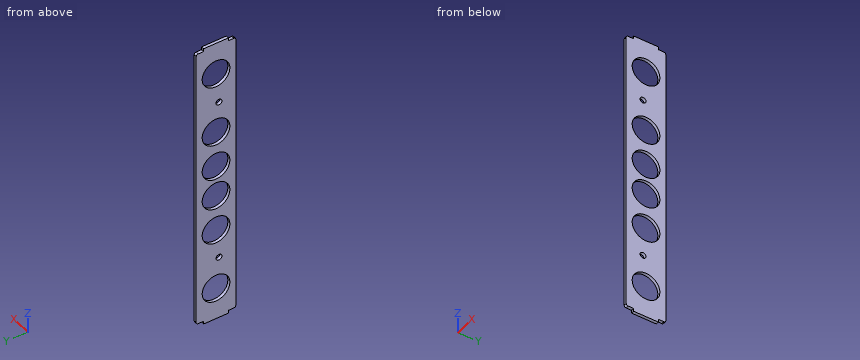
```python
from build123d import *

# Parameters (mm, degrees)
SKETCH3_W           = 292
SKETCH3_H           = 40
SKETCH3_R           = 3
BOSS_EXTRUDE2_DEPTH = 3
FILLET1_R           = 2
SKETCH4_R           = 14
CUT_EXTRUDE1_DEPTH  = 10
SKETCH5_W           = 3
SKETCH5_H           = 25
BOSS_EXTRUDE3_DEPTH = 3


with BuildPart() as part:
    # Sketch3 → Boss-Extrude2 (new body)
    with BuildSketch(Plane(origin=(0, 0, 0), x_dir=(0, 0, -1), z_dir=(1, 0, 0))):
        with Locations((146, -20)):
            Rectangle(SKETCH3_W, SKETCH3_H)
        with Locations((62, -23)):
            Circle(SKETCH3_R, mode=Mode.SUBTRACT)
        with Locations((230, -23)):
            Circle(SKETCH3_R, mode=Mode.SUBTRACT)
    extrude(amount=BOSS_EXTRUDE2_DEPTH)

    # Fillet1
    fillet1_edges = [part.edges().sort_by_distance(p)[0] for p in [
        (1.5, -40, -292),
        (1.5, -40, 0),
        (1.5, 0, 0),
        (1.5, 0, -292),
    ]]
    fillet(fillet1_edges, radius=FILLET1_R)

    # Sketch4 → Cut-Extrude1 (cut)
    with BuildSketch(Plane(origin=(3, 0, 0), x_dir=(0, 0, -1), z_dir=(1, 0, 0))):
        with Locations((30, -20)):
            Circle(SKETCH4_R)
        with Locations((93, -20)):
            Circle(SKETCH4_R)
        with Locations((130, -20)):
            Circle(SKETCH4_R)
        with Locations((162, -20)):
            Circle(SKETCH4_R)
        with Locations((199, -20)):
            Circle(SKETCH4_R)
        with Locations((262, -20)):
            Circle(SKETCH4_R)
    extrude(amount=-CUT_EXTRUDE1_DEPTH, mode=Mode.SUBTRACT)

    # Sketch5 → Boss-Extrude3 (add)
    with BuildSketch(Plane(origin=(3, 0, 0), x_dir=(0, 0, -1), z_dir=(1, 0, 0))):
        with Locations((-1.5, -20)):
            Rectangle(SKETCH5_W, SKETCH5_H)
        with Locations((293.5, -20)):
            Rectangle(SKETCH5_W, SKETCH5_H)
    extrude(amount=-BOSS_EXTRUDE3_DEPTH)


solid = part.part
```
The listing builds one solid part. Answer for the finished solid, in the listing's coordinates (mm). Coordinates: 2 decimals unless noted, no trailing zeros. Write each loop counter-clockwise with the first axis right and the second up, starting at its lowest first coordinate (ties: lowest second). Pieces come first, ordered by that corner, then holes. Notation, with made-up numbers: (29, 59) - (38, 59) arc R26 cw to (38, 76) - close; hole circle Ø10 at (79.5, 62.5). An arc over 180 degrees is marked (long way). Return JSON: item names as keys, results as strings. Group by question number.
1. Given pin 1 (5.5 mm diameter, centred on y = -23, z = -230, fed in from +X); pin 2 (1.5 mm diameter, centred on x = 1, y = -3.5, fed in from +Z); pin 3 (1.5 mm diameter, centred on x = 2, z = 1.5, fed in from -Y); pin 4 (0.9 mm diameter, centred on x = 1, y = -35.5, fed in from -Z), each flat-ended and moving along its own axis, determine where each tip first touches the part or whether it passes through.
2. Straight lines are drawn through the part: L1, parallel to Y at x = 1.75, z = -199; L2, parallel to Y at x = 1.7, z = -230; L3, parallel to Z at x = 1.5, y = -35. For each, find the intervals that lie inside material, in ascending order.
3. A cutting plane is placed at A-A, the plane z = -199. Determine the outline of the cut face in (x, y), plus the area to 3 significant figures.
4. A cutting plane is placed at D-D, the plane z = -62. Determine the outline of the cut face in (x, y).
5. A cutting plane is placed at C-C, the plane x = 1.8. Give the number of separate pieces and of enclosed holes in the cut face, plus the area to 3 significant figures.
6. A cutting plane is placed at B-B, the plane y = -15. Determine the outline of the cut face in (x, z).
Ans:
{
 "1": {"pin 1": "through", "pin 2": "z = 0", "pin 3": "y = -32.5", "pin 4": "z = -292"},
 "2": {"L1": "-40 to -34, -6 to 0", "L2": "-40 to -26, -20 to 0", "L3": "-292 to 0"},
 "3": {"outline": "(0, -40) - (3, -40) - (3, -34) - (0, -34) - close; (0, -6) - (3, -6) - (3, 0) - (0, 0) - close", "area": "36.0 mm²"},
 "4": {"outline": "(0, -40) - (3, -40) - (3, -26) - (0, -26) - close; (0, -20) - (3, -20) - (3, 0) - (0, 0) - close"},
 "5": {"separate pieces": "1", "enclosed holes": "8", "area": "8,080 mm²"},
 "6": {"outline": "(0, -295) - (3, -295) - (3, -275.08) - (0, -275.08) - close; (0, -248.92) - (3, -248.92) - (3, -212.08) - (0, -212.08) - close; (0, -185.92) - (3, -185.92) - (3, -175.08) - (0, -175.08) - close; (0, -148.92) - (3, -148.92) - (3, -143.08) - (0, -143.08) - close; (0, -116.92) - (3, -116.92) - (3, -106.08) - (0, -106.08) - close; (0, -79.92) - (3, -79.92) - (3, -43.08) - (0, -43.08) - close; (0, -16.92) - (3, -16.92) - (3, 3) - (0, 3) - close"}
}
